Answer from the drawing. Dimensions are ordinates in mm from the lowest x, y and z of the part. Give positions to 0.01 mm unless a question says otherwise; leave off trailing zeros. Loops run counter-clockwise (first coordinate to the right, second up) from the corner with the lowest first, then second, coordinate; pieces in that order, holes last. Notation, with made-up numbers: (43, 12.25) - (62, 12.25) arc R19 ccw to (62, 18.25) - close; hole circle Ø5 at (34, 52.25). An arc over 180 degrees is marked (long way). Put each result on its own line as item: value. Start each with the question number.
1. Given pin 1 Ø3 at (x, z) = (122, 120.5) entering from -Y; pin 2 Ø0.9 at (y, z) = (1, 34) entering from +X; pin 3 Ø0.9 at (y, z) = (1, 41.5) entering from -X; pin 4 Ø0.9 at (x, y) = (111.5, 2) entering from +Z, each flat-ended and moving along its own axis, determine where each tip first touches the part or whether it passes through.
2. Consider L1, parallel to X at y = 2.1, z = 113; L2, parallel to Z at x = 105.5, y = 1.55; L3, parallel to Z at x = 108, y = 0.55. Determine where each line is inside the solid, lowest interval first. Write a range as from..to.
3. A cutting plane is placed at A-A, the plane x = 120. Determine the outline of the cut face in (y, z), plus the area to 3 significant figures.
4. A cutting plane is placed at B-B, the plane z = 117.5. Determine the outline of the cut face in (x, y), plus the area to 3 significant figures.
5. A cutting plane is placed at C-C, the plane y = 0.65. Determine the outline of the cut face in (x, z).
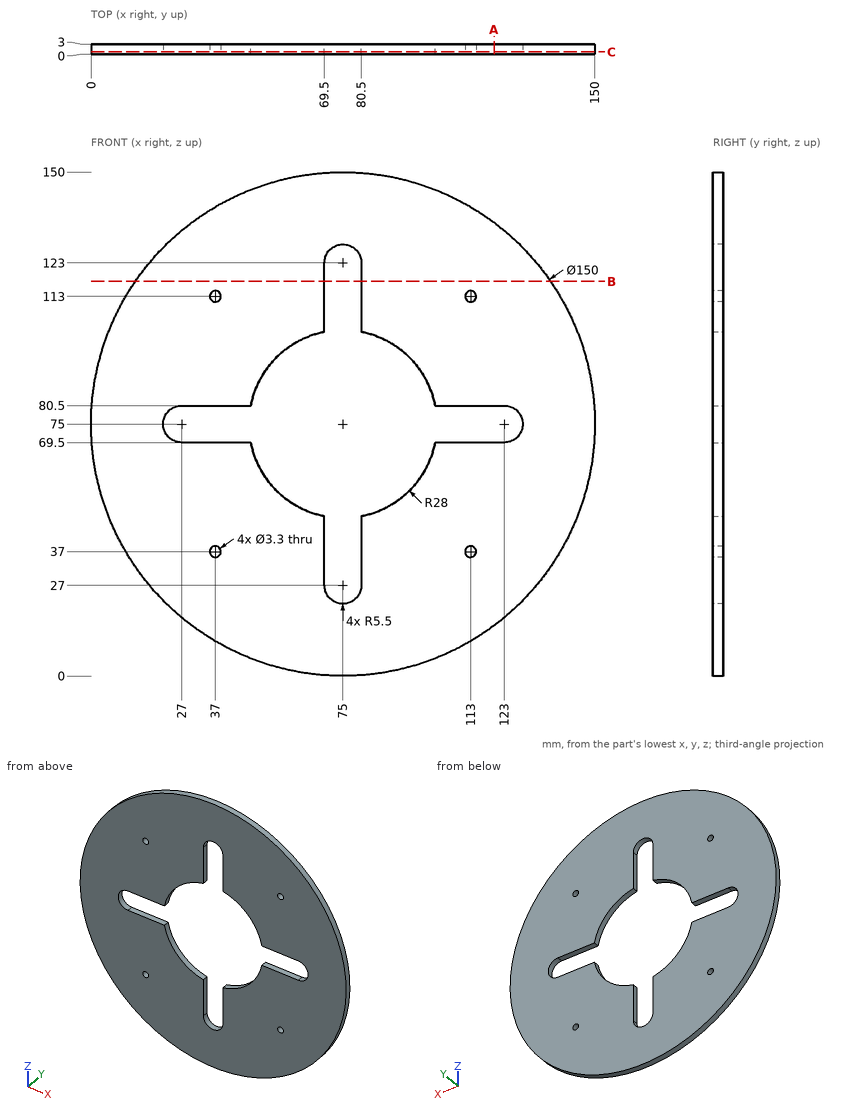
Return value:
1. pin 1: stops at y = 0
1. pin 2: stops at x = 138.09
1. pin 3: stops at x = 7.67
1. pin 4: stops at z = 140.77
2. L1: x = 10.34..35.35, 38.65..69.5, 80.5..111.35, 114.65..139.66
2. L2: z = 6.48..69.5, 80.5..143.52
2. L3: z = 7.65..69.5, 80.5..142.35
3. outline: (0, 15) - (3, 15) - (3, 69.5) - (0, 69.5) - close; (0, 80.5) - (3, 80.5) - (3, 135) - (0, 135) - close
3. area: 327 mm2
4. outline: (13.2, 0) - (69.5, 0) - (69.5, 3) - (13.2, 3) - close; (80.5, 0) - (136.8, 0) - (136.8, 3) - (80.5, 3) - close
4. area: 338 mm2
5. outline: circle Ø150 at (75, 75); hole (27, 69.5) - (47.55, 69.5) arc R28 ccw to (69.5, 47.55) - (69.5, 27) arc R5.5 ccw to (80.5, 27) - (80.5, 47.55) arc R28 ccw to (102.45, 69.5) - (123, 69.5) arc R5.5 ccw to (123, 80.5) - (102.45, 80.5) arc R28 ccw to (80.5, 102.45) - (80.5, 123) arc R5.5 ccw to (69.5, 123) - (69.5, 102.45) arc R28 ccw to (47.55, 80.5) - (27, 80.5) arc R5.5 ccw to start; hole circle Ø3.3 at (37, 37); hole circle Ø3.3 at (37, 113); hole circle Ø3.3 at (113, 37); hole circle Ø3.3 at (113, 113)
